For this review, use the dimensioned drawing (mm, ordinates from the lowest corner) and the shaded views. A direction names the side the tool comes from. Round coordinates to 2 decimals unless told otherwise and drop trailing zeros. Write each loop counter-clockwise with the first axis right and the second up, starting at its lowest first coordinate (ties: lowest second). Pieces come first, ordered by that corner, then holes. Notation, with made-up numbers: (73.25, 82) -> (82.25, 82) arc R8 ccw to (82.25, 97) -> close; hole circle Ø5 at (-31.5, 34.25). An arc over 180 degrees is marked (long way). Answer in a Markdown table with one row per item. Add a question column.
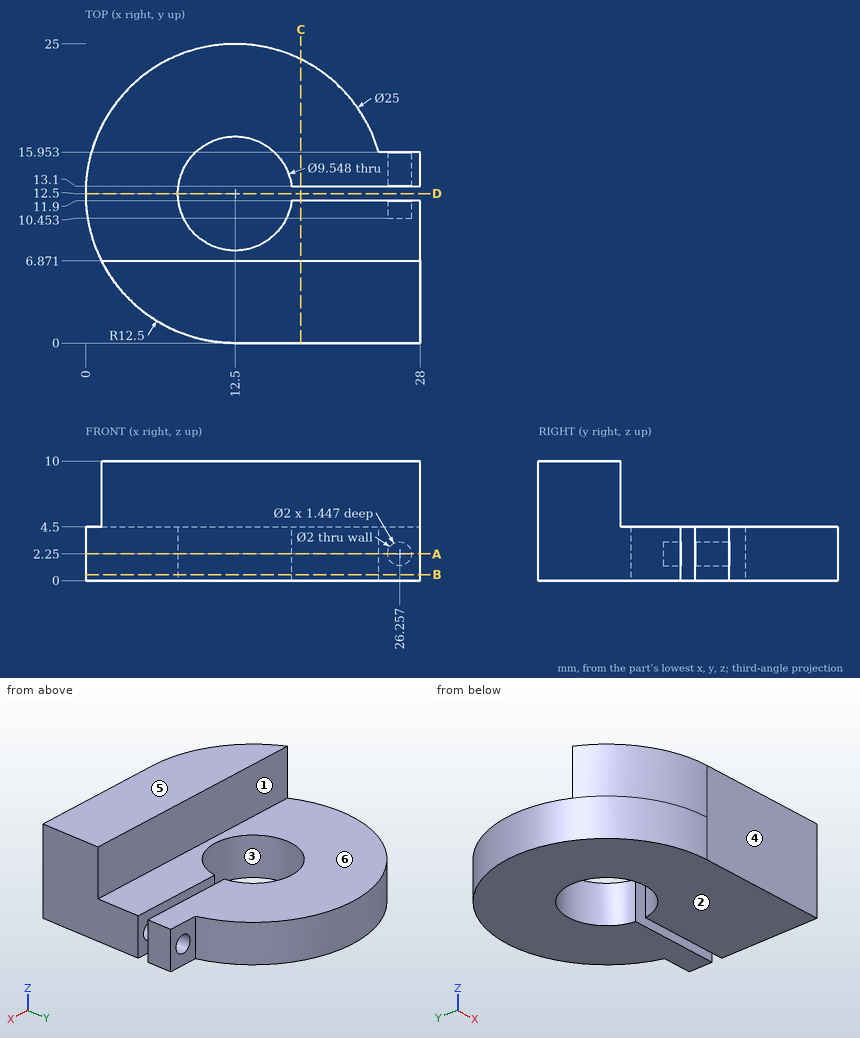
1. The part is to be moulded in two halves that separate along Y. For the marked faces 1, 2, 3 and 4, say which applies: pulls with the +Y half, pulls with the -Y half, needs draft (parallel to the pull), parting line crosses it, or undercut.
2. Tool access review of the marked faces 5 and 6: name each direction out of +Z, -Z, +X, -X, +Y, -Y from which nothing blocks a thin tool from reaching the whole face with its end or side.
3. For L1, parallel to Y at x = 12.5, z = 2.5; L2, parallel to Z at x = 18.75, y = 22.5; L3, parallel to X at y = 12.5, z = 3.3, list the stretches that pass through material, from the lowest coordinate up. Write a range as [from, to].
4. We need section C-C (x = 18). Write out the cut boundary in (y, z) (1 decimal), plus the area to 3 significant figures.
5. We need section B-B (z = 0.5). Write out the cut boundary in (x, y) (1 decimal), plus the area to 3 significant figures.
6. Clearance check with flat-ended pins moving along their axes: pin 1 Ø1 at (x, z) = (26.5, 1.5) entering from +Y; pin 2 Ø5.5 at (x, y) = (14, 18) entering from +Z; pin 3 Ø2 at (x, z) = (23, 3) entering from +Y (1 decimal). State where each tip first meets the part, or that it passes through.
7. We need section A-A (z = 2.25). Write out the cut boundary in (x, y) (1 decimal).
8. We need section D-D (y = 12.5). Write out the cut boundary in (x, z).
Response:
| question | item | result |
|---|---|---|
| 1 | face 1 | pulls with the +Y half |
| 1 | face 2 | needs draft |
| 1 | face 3 | undercut |
| 1 | face 4 | pulls with the -Y half |
| 2 | face 5 | +Z, +X, -X, +Y, -Y |
| 2 | face 6 | +Z, +X, -X, +Y |
| 3 | L1 | [0, 7.73], [17.27, 25] |
| 3 | L2 | [0, 4.5] |
| 3 | L3 | [0, 7.73] |
| 4 | outline | (0, 0) -> (11.9, 0) -> (11.9, 4.5) -> (6.9, 4.5) -> (6.9, 10) -> (0, 10) -> close; (13.1, 0) -> (23.7, 0) -> (23.7, 4.5) -> (13.1, 4.5) -> close |
| 4 | area | 139 mm2 |
| 5 | outline | (12.5, 0) -> (28, 0) -> (28, 11.9) -> (17.2, 11.9) arc R4.8 cw (long way) to (17.2, 13.1) -> (28, 13.1) -> (28, 16) -> (24.5, 16) arc R12.5 ccw (long way) to start |
| 5 | area | 488 mm2 |
| 6 | pin 1 | y = 15.95 |
| 6 | pin 2 | z = 4.5 |
| 6 | pin 3 | y = 20.6 |
| 7 | outline | (12.5, 0) -> (28, 0) -> (28, 11.9) -> (27.3, 11.9) -> (27.3, 10.5) -> (25.3, 10.5) -> (25.3, 11.9) -> (17.2, 11.9) arc R4.8 cw (long way) to (17.2, 13.1) -> (25.3, 13.1) -> (25.3, 16) -> (24.5, 16) arc R12.5 ccw (long way) to start; (27.3, 13.1) -> (28, 13.1) -> (28, 16) -> (27.3, 16) -> close |
| 8 | outline | (0, 0) -> (7.73, 0) -> (7.73, 4.5) -> (0, 4.5) -> close |
